```python
from build123d import *

# Parameters (mm, degrees)
F0_R     = 3
F1_DEPTH = 6
F3_DEPTH = 6
F4_R     = 5


with BuildPart() as f1:
    # F0 (on Right) → F1 (new body)
    with BuildSketch(Plane.YZ):
        Polygon((0, 63.333333), (-54.848276, -31.666667), (54.848276, -31.666667), align=None)
        with Locations((0, 53.333333)):
            Circle(F0_R, mode=Mode.SUBTRACT)
    extrude(amount=F1_DEPTH)

    # F2 (on face) → F3 (cut, through all)
    with BuildSketch(Plane.YZ.offset(6)):
        with BuildLine():
            ThreePointArc((23.244004, 3.486405), (0, -1.666667), (-23.244004, 3.486405))
            Line((-23.244004, 3.486405), (-31.69637, -14.639751))
            ThreePointArc((-31.69637, -14.639751), (0, -21.666667), (31.69637, -14.639751))
            Line((31.69637, -14.639751), (23.244004, 3.486405))
        make_face()
    extrude(amount=-F3_DEPTH, mode=Mode.SUBTRACT)

    # F4
    f4_edges = [f1.edges().sort_by_distance(p)[0] for p in [
        (3, 0, 63.333333),
    ]]
    fillet(f4_edges, radius=F4_R)


solid = f1.part
```
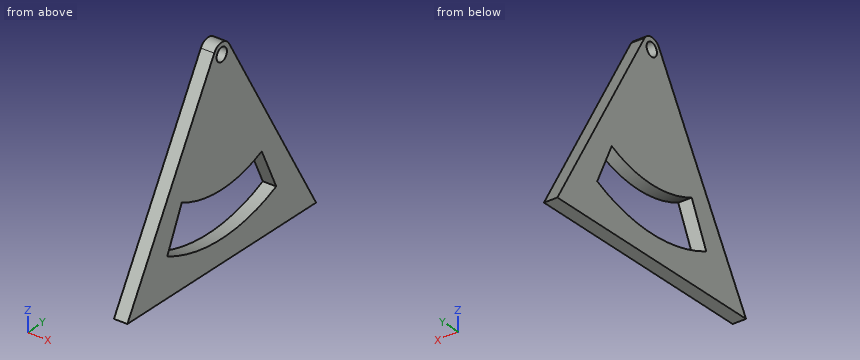
For this review, take the finished solid that the model builds, in its own axes (mm). Round coordinates to 2 decimals unless told otherwise and drop trailing zeros. Write each loop counter-clockwise with the first axis right and the second up, starting at its lowest first coordinate (ties: lowest second). Pieces come first, ordered by that corner, then holes. Notation, with made-up numbers: (55.5, 56) - (59.5, 56) arc R18 cw to (59.5, 91) - close; hole circle Ø6 at (-24, 50.25). An arc over 180 degrees is marked (long way). Answer as a JSON object with one key per item and string values.
1. To check wall thickness, follow line 1 along Y through (x, z) = (0.85, 3); line 2 along Z through (x, y) = (1.5, -5); line 3 along Z through (x, y) = (2.15, 26). State the ranges of each line that lie inside material, in increasing order.
Response values:
{"line 1": "y = -34.83 to -23.47, -22.17 to 22.17, 23.47 to 34.83", "line 2": "z = -31.67 to -21.5, -1.44 to 54.67", "line 3": "z = -31.67 to -17.02, -2.42 to 18.3"}
2. For pin 1 Ø3 at (x, y) = (3.5, 24.5) entering from +Z; pin 2 Ø2 at (x, z) = (3, 16) entering from +Y; pin 3 Ø10 at (y, z) = (0, -9) entering from -X; pin 4 Ø2 at (x, z) = (4, 40.5) entering from -Y, all flat-tipped, find the tip position at first contact; note any pin that passes through.
Response values:
{"pin 1": "stops at z = 23.5", "pin 2": "stops at y = 27.91", "pin 3": "passes through", "pin 4": "stops at y = -13.76"}
3. We need section C-C on x = 4.25. Give the boundary of the cut face in (y, z), then the cut area to 3 significant figures.
Response values:
{"outline": "(-54.85, -31.67) - (54.85, -31.67) - (4.33, 55.83) arc R5 ccw to (-4.33, 55.83) - close; hole (-31.7, -14.64) arc R75 ccw to (31.7, -14.64) - (23.24, 3.49) arc R55 cw to (-23.24, 3.49) - close; hole circle Ø6 at (0, 53.33)", "area": "4,030 mm2"}
4. We need section A-A on y = 0. Give the boundary of the cut face in (x, z).
Response values:
{"outline": "(0, -31.67) - (6, -31.67) - (6, -21.67) - (0, -21.67) - close; (0, -1.67) - (6, -1.67) - (6, 50.33) - (0, 50.33) - close; (0, 56.33) - (6, 56.33) - (6, 58.33) - (0, 58.33) - close"}
5. We need section B-B on z = -13.5. Give the boundary of the cut face in (x, y).
Response values:
{"outline": "(0, -44.36) - (6, -44.36) - (6, -31.16) - (0, -31.16) - close; (0, 31.16) - (6, 31.16) - (6, 44.36) - (0, 44.36) - close"}
6. We need section D-D on y = -15.5. Give the boundary of the cut face in (x, z), then the cut area to 3 significant figures.
Response values:
{"outline": "(0, -31.67) - (6, -31.67) - (6, -20.05) - (0, -20.05) - close; (0, 0.56) - (6, 0.56) - (6, 36.49) - (0, 36.49) - close", "area": "285 mm2"}
